Here's how the part is built. I have some questions about the finished solid (model axes, mm). Face numbers are marked on the shaded views. A direction names the side the tool comes from. Round coordinates to 2 decimals unless told otherwise and drop trailing zeros. Write each loop counter-clockwise with the first axis right and the second up, starting at its lowest first coordinate (ties: lowest second). Pieces come first, ordered by that corner, then holes. Notation, with made-up numbers: (53, -36.75) -> (92, -36.75) arc R15 cw to (92, -13.75) -> close; hole circle Ø7 at (-37, 69.25). An arc over 180 degrees is marked (long way). Put each result on its own line as item: value. Start each with the question number.
1) I want a section at D-D, the plane x = 4.75. List the corners of the cut face in (y, z) for me, then the cut area to 3 significant figures.
2) Which directions (+Z, -Z, +X, -X, +Y, -Y) give clear straight access to the entire face, cutting with the end or side of a thin tool? Please do the marked faces 4 and 5.
3) Will these pins go through, and if not, where does the flat tip stop? P1, Ø10, axis at y = -6.5, z = 22.5, coming from the +X side; P2, Ø2, axis at x = -7, z = 38, coming from the -Y side; P3, Ø10, axis at x = 5.5, z = 32.5, coming from the +Y side.
4) I want a section at A-A, the plane x = 0. List the corners of the cut face in (y, z) for me (3 decimals), then the cut area to 3 significant figures.
5) If I drill on line 1 along Y through (x, z) = (0, 5.75) (3 decimals); line 2 along Y through (x, z) = (0, 38) (3 decimals); line 3 along Z through (x, y) = (4.5, 2.75), over which ranges is the centre line in solid material (lowest first)? Write a range as [from, to].
6) We'd pull the mould along Y, two halves only. Please class the marked faces 1, 2 and 3: released by +Y, released by -Y, zero draft, split by the parting line, or undercut.
7) I want a section at C-C, the plane z = 49. List the corners of the cut face in (x, y) for me (3 decimals).
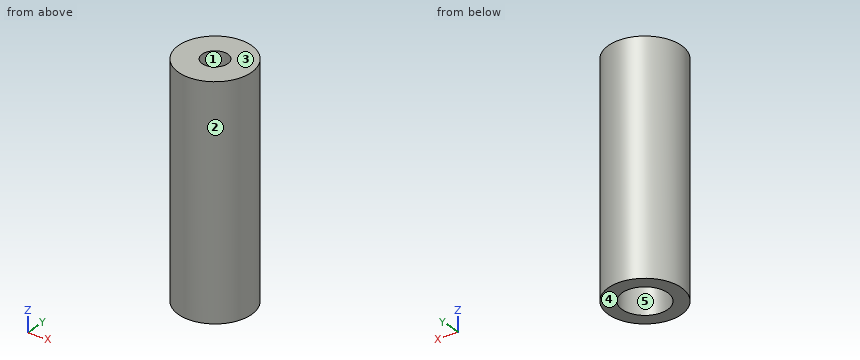
from build123d import *

# Parameters (mm, degrees)
ESBO_O1_R                = 9
RESSALTO_EXTRUS_O1_DEPTH = 56
ESBO_O2_R                = 5.615
CORTE_EXTRUS_O1_DEPTH    = 7.54
ESBO_O3_R                = 3.175
CORTE_EXTRUS_O2_DEPTH    = 49.46


with BuildPart() as part:
    # Esboço1 → Ressalto-extrusão1 (new body)
    with BuildSketch(Plane.XY):
        Circle(ESBO_O1_R)
    extrude(amount=RESSALTO_EXTRUS_O1_DEPTH)

    # Esboço2 → Corte-extrusão1 (cut)
    with BuildSketch(Plane(origin=(0, 0, 0), x_dir=(-1, 0, 0), z_dir=(0, 0, -1))):
        Circle(ESBO_O2_R)
    extrude(amount=-CORTE_EXTRUS_O1_DEPTH, mode=Mode.SUBTRACT)

    # Esboço3 → Corte-extrusão2 (cut, through all)
    with BuildSketch(Plane(origin=(0, 0, 7.54), x_dir=(-1, 0, 0), z_dir=(0, 0, -1))):
        Circle(ESBO_O3_R)
    extrude(amount=-CORTE_EXTRUS_O2_DEPTH, mode=Mode.SUBTRACT)


solid = part.part
Findings:
1. outline: (-7.64, 0) -> (-2.99, 0) -> (-2.99, 7.54) -> (2.99, 7.54) -> (2.99, 0) -> (7.64, 0) -> (7.64, 56) -> (-7.64, 56) -> close
1. area: 811 mm2
2. face 4: -Z, +X, -X, +Y, -Y
2. face 5: -Z
3. P1: stops at x = 8.87
3. P2: stops at y = -6.71
3. P3: stops at y = 8.99
4. outline: (-9, 0) -> (-5.615, 0) -> (-5.615, 7.54) -> (-3.175, 7.54) -> (-3.175, 56) -> (-9, 56) -> close; (3.175, 7.54) -> (5.615, 7.54) -> (5.615, 0) -> (9, 0) -> (9, 56) -> (3.175, 56) -> close
4. area: 616 mm2
5. line 1: y = [-9, -5.615], [5.615, 9]
5. line 2: y = [-9, -3.175], [3.175, 9]
5. line 3: z = [7.54, 56]
6. face 1: undercut
6. face 2: split by the parting line
6. face 3: zero draft
7. outline: circle Ø18 at (0, 0); hole circle Ø6.35 at (0, 0)
